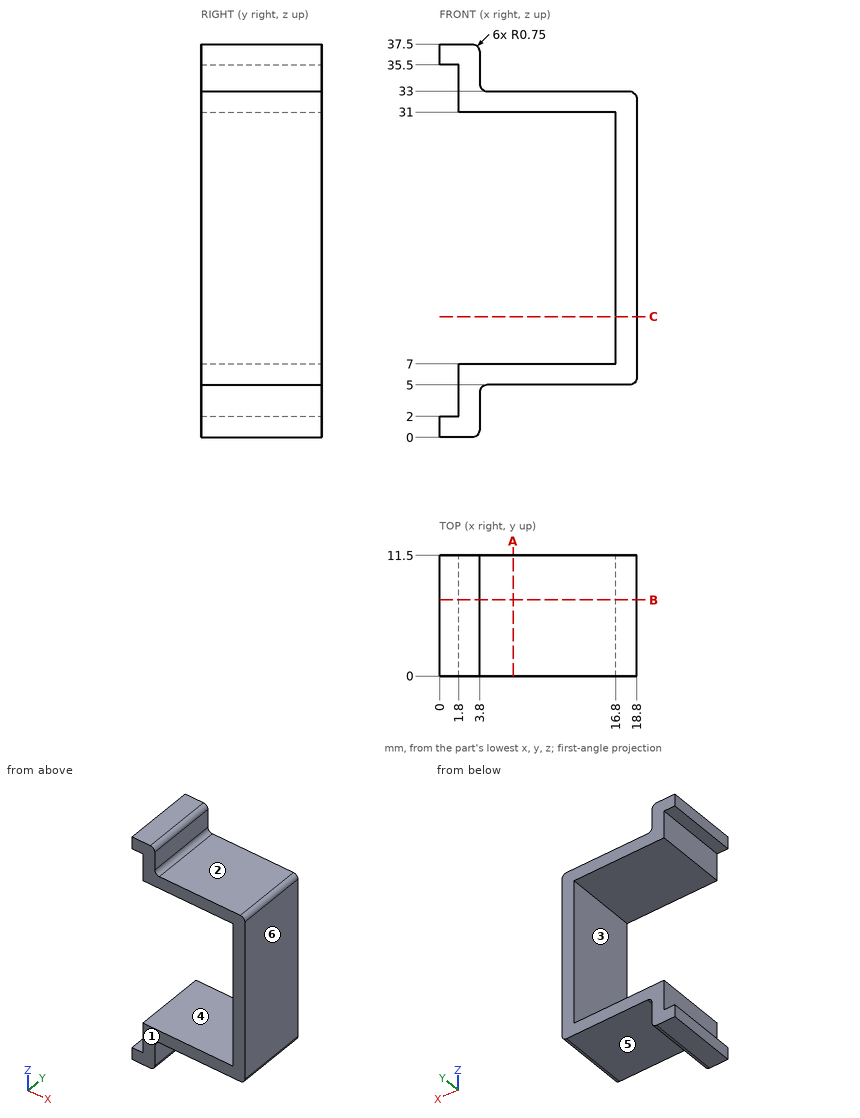
Geometry check sheet. Reference: drawing and pictorial views, mm from the part's lowest x, y, z. A direction names the side the tool comes from. Round coordinates to 2 decimals unless told otherwise and drop trailing zeros. Order: outer loops, then holes, each group sorted by start corner. A loop starts at its lowest first (then second) coordinate and runs counter-clockwise, first axis right, second up. Notation, with made-up numbers: (-9.5, 39.25) - (0.5, 39.25) arc R21 cw to (0.5, 67.25) - close; hole circle Ø10 at (89.5, 50). An arc over 180 degrees is marked (long way). Write item = value, one per line.
Q1. Section check B-B (y = 7.25). Record the boundary of the cut face in (x, z).
Computed:
outline = (0, 0) - (3.05, 0) arc R0.75 ccw to (3.8, 0.75) - (3.8, 4.25) arc R0.75 cw to (4.55, 5) - (18.05, 5) arc R0.75 ccw to (18.8, 5.75) - (18.8, 32.25) arc R0.75 ccw to (18.05, 33) - (4.55, 33) arc R0.75 cw to (3.8, 33.75) - (3.8, 36.75) arc R0.75 ccw to (3.05, 37.5) - (0, 37.5) - (0, 35.5) - (1.8, 35.5) - (1.8, 31) - (16.8, 31) - (16.8, 7) - (1.8, 7) - (1.8, 2) - (0, 2) - close
Q2. Draft check along Z on the marked faces 4, 5 and 6. Enter one of: pulls with the +Z half, pulls with the -Z half, needs draft (parallel to the pull), parting line crosses it, or undercut.
Computed:
face_4 = undercut
face_5 = pulls with the -Z half
face_6 = needs draft
Q3. Section check C-C (z = 11.5). Record the boundary of the cut face in (x, y), and give its area (3 significant figures).
Computed:
outline = (16.8, 0) - (18.8, 0) - (18.8, 11.5) - (16.8, 11.5) - close
area = 23.0 mm^2
Q4. Thickness scan on line 1 along Z through (x, y) = (16.75, 10.25); line 2 along Z through (x, y) = (2.25, 4.5); line 3 along X through (y, z) = (1.75, 10). Record the ranges inside material, lowest first.
Computed:
line_1 = 5 to 7, 31 to 33
line_2 = 0 to 7, 31 to 37.5
line_3 = 16.8 to 18.8
Q5. Tool access check on the marked faces 1, 2 and 3. Record the directions out of +Z, -Z, +X, -X, +Y, -Y that give a thin tool (end or side, any length) a straight path to the whole face; none if there is none.
Computed:
face_1 = +Z, -Z, +X, -X, -Y
face_2 = +Z, +X, +Y, -Y
face_3 = -X, +Y, -Y
Q6. Go/stop test with flat-tipped pins: pin 1 (3 mm diameter, centred on y = 3.5, z = 10.5, fed in from -X); pin 2 (2.5 mm diameter, centred on y = 8, z = 4, fed in from -X); pin 3 (3 mm diameter, centred on x = 8, y = 7, fed in from +Z). Record where each tip stops, or that it passes through.
Computed:
pin_1 = 16.8
pin_2 = 1.8
pin_3 = 33
Q7. Section check A-A (x = 7). Record the boundary of the cut face in (y, z), and give its area (3 significant figures).
Computed:
outline = (0, 5) - (11.5, 5) - (11.5, 7) - (0, 7) - close; (0, 31) - (11.5, 31) - (11.5, 33) - (0, 33) - close
area = 46.0 mm^2
